Work out the finished part from the listing and answer in its coordinate system (mm). A direction names the side the tool comes from. Round coordinates to 2 decimals unless told otherwise and drop trailing zeros. Order: outer loops, then holes, each group sorted by start corner. A loop starts at its lowest first (then second) coordinate and runs counter-clockwise, first axis right, second up. Notation, with made-up numbers: (18, -39) - (45, -39) arc R12 cw to (45, -25) - close; hole circle Ø10 at (-37, -12). An arc over 180 degrees is marked (long way). Answer in a Markdown table with one row per item.
from build123d import *

# Parameters (mm, degrees)
EXTRUDE_1_DEPTH     = 8
FILLET_1_R          = 1
CUT_EXTRUDE_1_DEPTH = 36
FILLET_2_R          = 1


with BuildPart() as part:
    # 스케치1 → 보스-돌출1 (new body)
    with BuildSketch(Plane.XY):
        Polygon((21, 50), (21, -50), (-21, -50), align=None)
    extrude(amount=EXTRUDE_1_DEPTH)

    # 필렛1
    fillet_1_edges = [part.edges().sort_by_distance(p)[0] for p in [
        (21, -50, 4),
        (-21, -50, 4),
        (21, 50, 4),
    ]]
    fillet(fillet_1_edges, radius=FILLET_1_R)

    # 스케치2 → 컷-돌출1 (cut)
    with BuildSketch(Plane.XY.offset(8)):
        Polygon((13, -42), (13, 10.292957161), (-8.963042008, -42), align=None)
    extrude(amount=-CUT_EXTRUDE_1_DEPTH, mode=Mode.SUBTRACT)

    # 필렛2
    fillet_2_edges = [part.edges().sort_by_distance(p)[0] for p in [
        (13, 10.292957161, 4),
        (13, -42, 4),
        (-8.963042008, -42, 4),
    ]]
    fillet(fillet_2_edges, radius=FILLET_2_R)


solid = part.part
1) Find section A-A, the plane z = 2.5. Give the vertices of the cut face in (x, y), then the cut area to 3 significant figures.
Filled in:
| item | result |
|---|---|
| outline | (-20.42, -48.61) arc R1 ccw to (-19.5, -50) - (20, -50) arc R1 ccw to (21, -49) - (21, 45.04) arc R1 ccw to (19.08, 45.42) - close; hole (-8.38, -40.61) arc R1 ccw to (-7.46, -42) - (12, -42) arc R1 ccw to (13, -41) - (13, 5.33) arc R1 ccw to (11.08, 5.72) - close |
| area | 1,530 mm^2 |
2) Find section B-B, the plane x = 1. Give the vertices of the cut face in (y, z).
Filled in:
| item | result |
|---|---|
| outline | (-50, 0) - (-42, 0) - (-42, 8) - (-50, 8) - close; (-18.28, 0) - (2.38, 0) - (2.38, 8) - (-18.28, 8) - close |
3) Find the intervals of material crossed by probe 1 along Y at (x, z) = (2.5, 4); probe 2 along Y at (x, z) = (-3, 7.25); probe 3 along X at (y, z) = (-11, 1.5), in increasing order. Write a range as from..to.
Filled in:
| item | result |
|---|---|
| probe 1 | y = -50..-42, -14.71..5.95 |
| probe 2 | y = -50..-42, -27.8..-7.14 |
| probe 3 | x = -4.62..4.06, 13..21 |
4) This flat-tipped pin is pushed along its axis until it touches: pin 1 (3 mm diameter, centred on x = 16.5, z = 4, fed in from +Y). Where does it stop, or does it pass through?
Filled in:
| item | result |
|---|---|
| pin 1 | stops at y = 42.86 |
5) Which of the six approach directions +Z, -Z, +X, -X, +Y, -Y give full straight-line access (tool end or side, diameter ignored) to faces 4 (the face through (1.485, -17.124, 4.056)), 5 (the face through (21, -1, 4))?
Filled in:
| item | result |
|---|---|
| face 4 | +Z, -Z |
| face 5 | +Z, -Z, +X, +Y, -Y |
6) The mould has two halves that part along X. Classify faces 1 (the face through (2, -42, 4)), 2 (the face through (1, -12, 8)), 3 (the face through (20.216, 46.013, 4.056)): released by +X, released by -X, zero draft, split by the parting line, or undercut.
Filled in:
| item | result |
|---|---|
| face 1 | undercut |
| face 2 | zero draft |
| face 3 | split by the parting line |
7) Find section D-D, the plane x = -14.5. Give the vertices of the cut face in (y, z), then the cut area to 3 significant figures.
Filled in:
| item | result |
|---|---|
| outline | (-50, 0) - (-34.52, 0) - (-34.52, 8) - (-50, 8) - close |
| area | 124 mm^2 |
8) Find section C-C, the plane y = -43. Give the vertices of the cut face in (x, z).
Filled in:
| item | result |
|---|---|
| outline | (-18.06, 0) - (21, 0) - (21, 8) - (-18.06, 8) - close |
